Geometry: final body of the model. Coordinates: model frame, mm. Give positions to 0.01 mm unless a question says otherwise; leave off trailing zeros. Order: outer loops, then holes, each group sorted by start corner. A loop starts at its lowest first (then second) coordinate and runs counter-clockwise, first axis right, second up. Notation, with made-up numbers: (16, 80.5) -> (63, 80.5) arc R31 cw to (63, 116.5) -> close; hole circle Ø7 at (-28.75, 87). An arc over 180 degrees is marked (long way). One line per question, with ' | ' between items. Start each with the question number.
(1) Section C-C (x = 18). Return loops of the section in (y, z).
(2) Section B-B (x = -32). Return loops of the section in (y, z).
(3) Section A-A (y = 1.2). Return loops of the section in (x, z), then the cut area to 3 significant figures.
(4) First-contact query: pin 1 Ø1.5 at (x, y) = (-48.5, 1) entering from -Z. Flat tip, straight axial feed; report the tip coordinate or a pass-through.
(5) Ray query, L1, parallel to X at y = 1.9, z = 99; L2, parallel to X at y = 0.55, z = -117.5; L3, parallel to Z at x = -43, y = 2.25. Return the intervals inside material, ascending.
```python
from build123d import *

# Parameters (mm, degrees)
SKETCH2_R           = 1.5
BOSS_EXTRUDE2_DEPTH = 2.6


with BuildPart() as part:
    # Sketch2 → Boss-Extrude2 (new body)
    with BuildSketch(Plane(origin=(0, 0, 0), x_dir=(1, 0, 0), z_dir=(0, 1, 0))):
        with BuildLine():
            Line((-80, -45), (-80, 45))
            ThreePointArc((-80, 45), (0, 125), (80, 45))
            Line((80, 45), (80, -45))
            ThreePointArc((80, -45), (0, -125), (-80, -45))
        make_face()
        with Locations(Location((14, 117.5, 0), (0, 0, 270))):
            Circle(SKETCH2_R, mode=Mode.SUBTRACT)
        with Locations(Location((14, 95.5, 0), (0, 0, 270))):
            Circle(SKETCH2_R, mode=Mode.SUBTRACT)
        with Locations(Location((-14, 95.5, 0), (0, 0, 270))):
            Circle(SKETCH2_R, mode=Mode.SUBTRACT)
        with Locations(Location((-14, 117.5, 0), (0, 0, 270))):
            Circle(SKETCH2_R, mode=Mode.SUBTRACT)
        with Locations(Location((42, -99, 0), (0, 0, 270))):
            Circle(SKETCH2_R, mode=Mode.SUBTRACT)
        with Locations(Location((-42, -99, 0), (0, 0, 270))):
            Circle(SKETCH2_R, mode=Mode.SUBTRACT)
    extrude(amount=BOSS_EXTRUDE2_DEPTH)


solid = part.part
```
Response:
1) outline: (0, -122.95) -> (2.6, -122.95) -> (2.6, 122.95) -> (0, 122.95) -> close
2) outline: (0, -118.32) -> (2.6, -118.32) -> (2.6, 118.32) -> (0, 118.32) -> close
3) outline: (-80, -45) arc R80 ccw to (80, -45) -> (80, 45) arc R80 ccw to (-80, 45) -> close; hole circle Ø3 at (-42, 99); hole circle Ø3 at (-14, -117.5); hole circle Ø3 at (-14, -95.5); hole circle Ø3 at (14, -117.5); hole circle Ø3 at (14, -95.5); hole circle Ø3 at (42, 99) | area: 34,500 mm^2
4) pin 1: stops at z = -109.19
5) L1: x = -59.03 to -43.5, -40.5 to 40.5, 43.5 to 59.03 | L2: x = -33.82 to -15.5, -12.5 to 12.5, 15.5 to 33.82 | L3: z = -112.46 to 97.88, 100.12 to 112.46
